For this review, take the finished solid that the model builds, in its own axes (mm). A direction names the side the tool comes from. Coordinates: 2 decimals unless noted, no trailing zeros. Loops run counter-clockwise (first coordinate to the right, second up) from the corner with the lowest first, then second, coordinate; pieces in that order, holes last. Notation, with made-up numbers: (84, -39.5) - (139, -39.5) arc R26 cw to (139, -15.5) - close; hole circle Ø5 at (29.5, 34.25). An arc over 180 degrees is marked (long way). Use one line per item in the form item = value. Start each with the question number.
1. Add section A-A on y = 0. Give the boundary of the cut face in (x, z), and give its area (3 significant figures).
2. To check wall thickness, follow probe 1 along Y at (x, z) = (0, 0.7); probe 2 along Y at (x, z) = (-1.5, 0.9); probe 3 along Z at (x, y) = (-1, 0.75). State the ranges of each line that lie inside material, in increasing order.
3. Draft analysis for pull direction X (two halves, no side actions). For faces 3 (the face through (-1.172, 8.923, 0.495)), 4 (the face through (-1.216, 1.115, 0.803)), 5 (the face through (2, 0, 1)), state which applies: +X half, -X half, draft (parallel to the pull), parting line (faces both ways), or undercut.
4. Machinability: for faces 1 (the face through (0, 0, 0.6)), 2 (the face through (0, 0, 0)), which of the approach directions +Z, -Z, +X, -X, +Y, -Y give a long, thin tool a straight path to every point of the face, cutting with its end or side? Answer none if there is none.
```python
from build123d import *

# Parameters (mm, degrees)
F0_R     = 9
F1_DEPTH = 1
F2_R     = 0.15
F3_R     = 1.65
F4_DEPTH = 0.4


# Not quite as in the source:
# - a feature names something its author has since deleted; it is built from what else it names


with BuildPart() as f1:
    # F0 (on Top) → F1 (new body)
    with BuildSketch(Plane.XY):
        Circle(F0_R)
    extrude(amount=F1_DEPTH)

    # F2
    f2_edges = [f1.edges().sort_by_distance(p)[0] for p in [
        (-9, 0, 1),
        (-9, 0, 0),
    ]]
    fillet(f2_edges, radius=F2_R)

    # F3 (on face) → F4 (cut)
    with BuildSketch(Plane.XY.offset(1)):
        Circle(F3_R)
    extrude(amount=-F4_DEPTH, mode=Mode.SUBTRACT)


solid = f1.part
```
Conclusion:
q1.outline = (-9, 0.15) arc R0.15 ccw to (-8.85, 0) - (8.85, 0) arc R0.15 ccw to (9, 0.15) - (9, 0.85) arc R0.15 ccw to (8.85, 1) - (1.65, 1) - (1.65, 0.6) - (-1.65, 0.6) - (-1.65, 1) - (-8.85, 1) arc R0.15 ccw to (-9, 0.85) - close
q1.area = 16.7 mm^2
q2.probe_1 = -9 to -1.65, 1.65 to 9
q2.probe_2 = -8.87 to -0.69, 0.69 to 8.87
q2.probe_3 = 0 to 0.6
q3.face_3 = parting line
q3.face_4 = undercut
q3.face_5 = draft
q4.face_1 = +Z
q4.face_2 = -Z, +X, -X, +Y, -Y
